Here's the drawing with two shaded views (mm, measured from the low corner). I have some questions. A direction names the side the tool comes from. Give positions to 0.01 mm unless a question says otherwise; leave off trailing zeros. Loops run counter-clockwise (first coordinate to the right, second up) from the corner with the lowest first, then second, coordinate; pieces in that order, holes last. Notation, with made-up numbers: M 65,70 L 83,70 A26 ccw 83,109 Z; hole C 44.25,25.25 d1. An arc over 180 degrees is marked long. Answer in a Markdown table with one row per item. Add a question column.
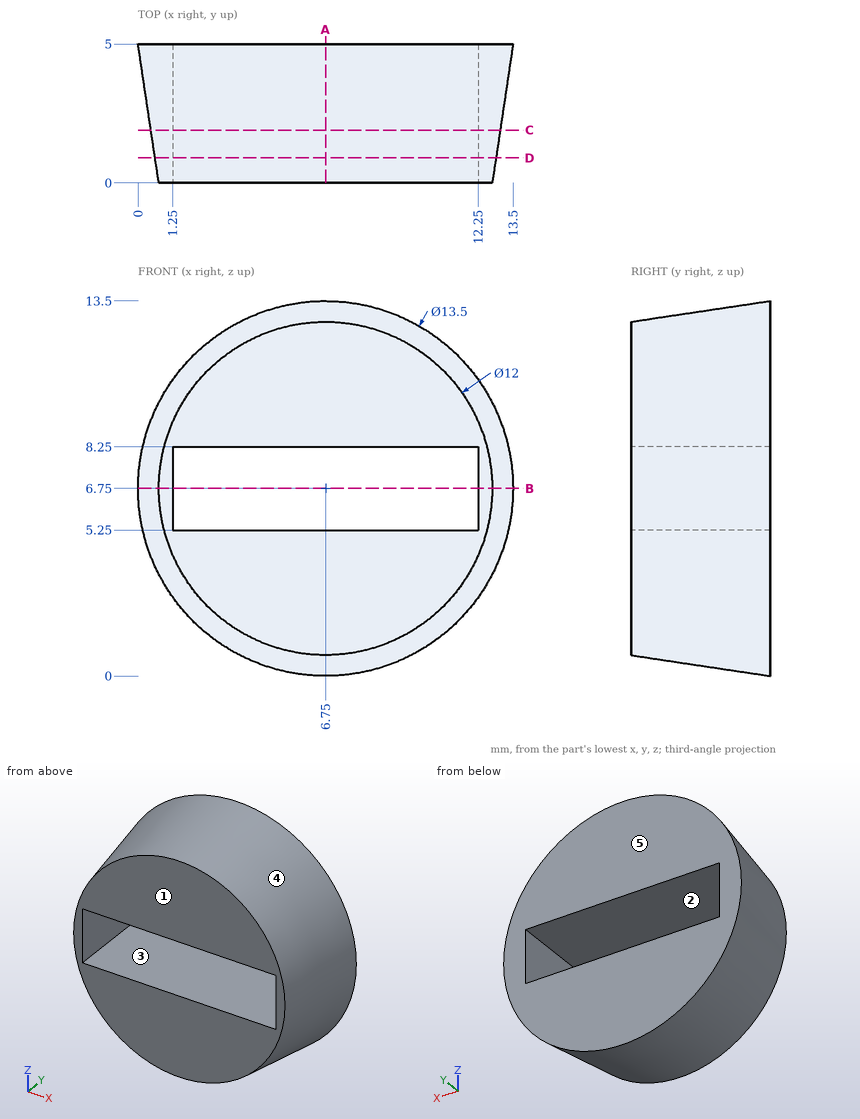
Item 1: If we mould it in two halves opening along X, with no side actions, what happens to the marked faces 3, 4 and 5? For each: +X half, -X half, draft (parallel to the pull), parting line (faces both ways), or undercut.
Item 2: Suppose I cut it at C-C (y = 1.9). List the corners of the cut face in (x, z) for me (3 decimals).
Item 3: For P1, Ø1.5, axis at x = 6, y = 2, coming from the +Z side; P2, Ø0.9, axis at y = 2, z = 7.5, coming from the +X side; P3, Ø1, axis at x = 2, y = 3, coming from the -Z side, each with a flat end and sliding along its axis, tell me the tip position at first contact or that it passes through.
Item 4: Suppose I cut it at B-B (z = 6.75). List the corners of the cut face in (x, y) for me.
Item 5: I need wall thicknesses on L1, parallel to Z at x = 8.75, y = 2.8; L2, parallel to Z at x = 11, y = 3.1; L3, parallel to X at y = 1.9, z = 6. Which ranges of each line are inside material? Lowest first, please.
Item 6: For the marked faces 1 and 2, which set-ups out of +Z, -Z, +X, -X, +Y, -Y let a thin tool reach every point of the face, with its end or its side?
Item 7: Suppose I cut it at A-A (x = 6.75). List the corners of the cut face in (y, z) for me.
Item 8: Suppose I cut it at D-D (y = 0.9). List the corners of the cut face in (x, z) for me (3 decimals).
Values found:
| question | item | result |
|---|---|---|
| 1 | face 3 | undercut |
| 1 | face 4 | parting line |
| 1 | face 5 | draft |
| 2 | outline | C 6.75,6.75 d12.57; hole M 1.25,5.25 L 12.25,5.25 L 12.25,8.25 L 1.25,8.25 Z |
| 3 | P1 | z = 13.14 |
| 3 | P2 | x = 13.09 |
| 3 | P3 | z = 1.89 |
| 4 | outline | M 0,5 L 0.75,0 L 1.25,0 L 1.25,5 Z; M 12.25,0 L 12.75,0 L 13.5,5 L 12.25,5 Z |
| 5 | L1 | 0.65 to 5.25, 8.25 to 12.85 |
| 5 | L2 | 1.88 to 5.25, 8.25 to 11.62 |
| 5 | L3 | 0.51 to 1.25, 12.25 to 12.99 |
| 6 | face 1 | +Z, -Z, +X, -X, -Y |
| 6 | face 2 | +Y, -Y |
| 7 | outline | M 0,0.75 L 5,0 L 5,5.25 L 0,5.25 Z; M 0,8.25 L 5,8.25 L 5,13.5 L 0,12.75 Z |
| 8 | outline | C 6.75,6.75 d12.27; hole M 1.25,5.25 L 12.25,5.25 L 12.25,8.25 L 1.25,8.25 Z |
